```python
from build123d import *

# Parameters (mm, degrees)
SKETCH_1_W                = 24
SKETCH_1_H                = 13.8
EXTRUDE_1_DEPTH           = 3.5
HOLE_WIZARD_1_D           = 3.4
HOLE_WIZARD_1_CBORE_D     = 6
HOLE_WIZARD_1_CBORE_DEPTH = 9
CUT_EXTRUDE_1_DEPTH       = 2
SKETCH_5_W                = 11
SKETCH_5_H                = 2.6
SKETCH_5_H_2              = 3
CUT_EXTRUDE_2_DEPTH       = 16.511608556
SKETCH_6_W                = 2
SKETCH_6_H                = 6
CUT_EXTRUDE_3_DEPTH       = 1
CHAMFER_1_SIZE            = 3.5
CHAMFER_2_SIZE            = 0.2
CHAMFER_3_SIZE            = 1


with BuildPart() as part:
    # 草图1 → 凸台-拉伸1 (new, symmetric)
    with BuildSketch(Plane.XY):
        Rectangle(SKETCH_1_W, SKETCH_1_H)
    extrude(amount=EXTRUDE_1_DEPTH, both=True)

    # 打孔尺寸根据内六角圆柱头螺钉的类型1 (through all)
    with Locations(Plane(origin=(0, 6.9, 0), x_dir=(1, 0, 0), z_dir=(0, 1, 0))):
        with Locations((4, 0), (-4, 0)):
            CounterBoreHole(HOLE_WIZARD_1_D / 2, HOLE_WIZARD_1_CBORE_D / 2, HOLE_WIZARD_1_CBORE_DEPTH)

    # 草图4 → 切除-拉伸1 (cut)
    with BuildSketch(Plane(origin=(0, 6.9, 0), x_dir=(1, 0, 0), z_dir=(0, 1, 0))):
        Polygon((9, 3.5), (6.979274058, 0), (9, -3.5), (12, -3.5), (12, 3.5), align=None)
    extrude(amount=-CUT_EXTRUDE_1_DEPTH, mode=Mode.SUBTRACT)

    # 草图5 → 切除-拉伸2 (cut, through all)
    with BuildSketch(Plane.XY.offset(3.5)):
        with Locations((6.5, -5.6)):
            Rectangle(SKETCH_5_W, SKETCH_5_H)
        with Locations((-6.5, -5.6)):
            Rectangle(SKETCH_5_W, SKETCH_5_H)
        with Locations((-6.5, 5.4)):
            Rectangle(SKETCH_5_W, SKETCH_5_H_2)
    extrude(amount=-CUT_EXTRUDE_2_DEPTH, mode=Mode.SUBTRACT)

    # 草图6 → 切除-拉伸3 (cut)
    with BuildSketch(Plane.XZ.offset(6.9)):
        Rectangle(SKETCH_6_W, SKETCH_6_H)
    extrude(amount=-CUT_EXTRUDE_3_DEPTH, mode=Mode.SUBTRACT)

    # 倒角1
    chamfer_1_edges = [part.edges().sort_by_distance(p)[0] for p in [
        (-12, -0.2, -3.5),
        (-12, -0.2, 3.5),
    ]]
    chamfer(chamfer_1_edges, length=CHAMFER_1_SIZE - 0.0001)  # a hair under: the kernel refuses the full size

    # 倒角2
    chamfer_2_edges = [part.edges().sort_by_distance(p)[0] for p in [
        (4, 6.9, -3.5),
        (4, 6.9, 3.5),
        (7.999894775, 6.9, 1.767766937),
        (7.999894775, 6.9, -1.767766937),
        (-1, 6.9, 0),
    ]]
    chamfer(chamfer_2_edges, length=CHAMFER_2_SIZE)

    # 倒角3
    chamfer_3_edges = [part.edges().sort_by_distance(p)[0] for p in [
        (12, 0.3, -3.5),
        (12, 0.3, 3.5),
    ]]
    chamfer(chamfer_3_edges, length=CHAMFER_3_SIZE)


solid = part.part
```
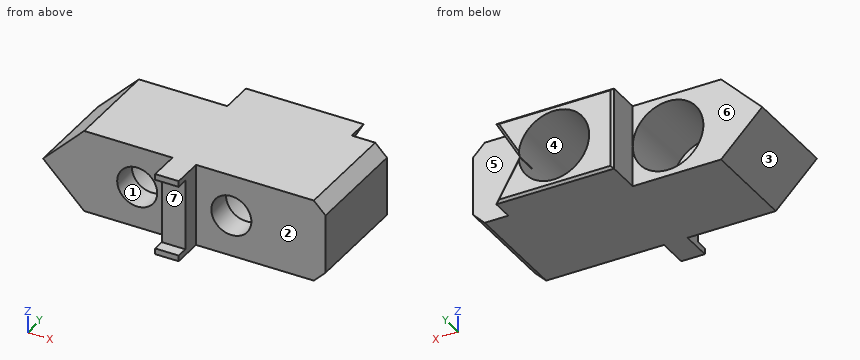
The model under review builds one solid part; all positions refer to its coordinate system, in mm. Face numbers are marked on the shaded views. A direction names the side the tool comes from. Coordinates: 2 decimals unless noted, no trailing zeros. Order: outer loops, then holes, each group sorted by start corner. A loop starts at its lowest first (then second) coordinate and runs counter-clockwise, first axis right, second up. Notation, with made-up numbers: M 49,13.5 L 102,13.5 A9 ccw 102,21.5 Z; hole C 51,37.5 d6. An arc over 180 degrees is marked long. One line per question, with ' | ' between items.
(1) The part is to be moulded in two halves that separate along Z. For the marked faces 1, 2 and 3, say which applies: +Z half, -Z half, draft (parallel to the pull), parting line (faces both ways), or undercut.
Geometry results:
face 1: undercut | face 2: draft | face 3: -Z half
(2) Add section A-A, the plane x = 4. Write out the cut boundary in (y, z), then the cut area to 3 significant figures.
Geometry results:
outline: M -4.3,-3.5 L 6.7,-3.5 L 6.9,-3.3 L 6.9,-3 L -2.1,-3 L -2.1,-1.7 L -4.3,-1.7 Z; M -4.3,1.7 L -2.1,1.7 L -2.1,3 L 6.9,3 L 6.9,3.3 L 6.7,3.5 L -4.3,3.5 Z | area: 16.9 mm²
(3) Add section B-B, the plane y = -3.5. State how many separate pieces and enclosed holes the cut face has, then the cut area to 3 significant figures.
Geometry results:
separate pieces: 1 | enclosed holes: 2 | area: 137 mm²
(4) Machinability: for the marked faces 4, 5, 6 and 7, which of the approach directions +Z, -Z, +X, -X, +Y, -Y give a long, thin tool a straight path to every point of the face, cutting with its end or side? Answer none if there is none.
Geometry results:
face 4: +Y | face 5: +X, +Y | face 6: +Z, -Z, -X, +Y | face 7: +X, -X, -Y
(5) Insertion check: pin 1 (0.8 mm diameter, centred on y = -6, z = -1.5, fed in from +X); pin 2 (0.8 mm diameter, centred on y = 5, z = 0, fed in from -X); pin 3 (2.5 mm diameter, centred on x = 4, z = 0, fed in from +Y); pin 4 (4 mm diameter, centred on x = -4, z = 0, fed in from +Y). Each pin has a flat end and moves straight along its axis. Give the tip position at first contact, or say it passes through.
Geometry results:
pin 1: stops at x = 1 | pin 2: stops at x = -1 | pin 3: passes through | pin 4: stops at y = -2.1
(6) For probe 1 along Z at (x, y) = (4, 0); probe 2 along X at (y, z) = (0.5, -1.5); probe 3 along Z at (x, y) = (-4, -3.3), list the stretches that pass through material, from the lowest coordinate up. Write a range as from..to.
Geometry results:
probe 1: z = -3.5..-3, 3..3.5 | probe 2: x = -10.5..-6.6, -1.4..1.4, 6.6..12 | probe 3: z = -3.5..-1.7, 1.7..3.5
(7) Add section D-D, the plane x = -4. Write out the cut boundary in (y, z).
Geometry results:
outline: M -4.3,-3.5 L 3.9,-3.5 L 3.9,-3 L -2.1,-3 L -2.1,-1.7 L -4.3,-1.7 Z; M -4.3,1.7 L -2.1,1.7 L -2.1,3 L 3.9,3 L 3.9,3.5 L -4.3,3.5 Z
